```python
from build123d import *

# Parameters (mm, degrees)
EXTRUDE_1_DEPTH     = 50
SKETCH_2_R          = 2
CUT_EXTRUDE_1_DEPTH = 51.670109532


with BuildPart() as part:
    # Эскиз1 → Бобышка-Вытянуть1 (new body)
    with BuildSketch(Plane.XY):
        with BuildLine():
            Line((-3.05, 2.308700651), (-3.05, -4.308700651))
            ThreePointArc((-3.05, -4.308700651), (0, -5.5), (3.05, -4.308700651))
            Line((3.05, -4.308700651), (3.05, 2.308700651))
            ThreePointArc((3.05, 2.308700651), (0, 3.5), (-3.05, 2.308700651))
        make_face()
    extrude(amount=EXTRUDE_1_DEPTH)

    # Эскиз2 → Вырез-Вытянуть1 (cut, through all)
    with BuildSketch(Plane.ZY.offset(3.05)):
        with Locations(Location((46, -1, 0), (0, 0, 270))):
            Circle(SKETCH_2_R)
    extrude(amount=-CUT_EXTRUDE_1_DEPTH, mode=Mode.SUBTRACT)


solid = part.part
```
Design review of the part built by this model. Coordinates are the model's own, in mm. Coordinates: 2 decimals unless noted, no trailing zeros. Write each loop counter-clockwise with the first axis right and the second up, starting at its lowest first coordinate (ties: lowest second). Pieces come first, ordered by that corner, then holes.
1) Insertion check: pin 1 (2 mm diameter, centred on x = 1, z = 11.5, fed in from +Y). The pin has a flat end and moves straight along its axis. Give the tip position at first contact, or say it passes through.
2) Mouldability with a two-part tool opening along Z and no side actions: class faces 1 (the flat face through (0, -1, 50)), 2 (the cylindrical face through (0, -5.5, 24.6)), 3 (the cylindrical face through (-0.043, -1.923, 44.226)) as +Z half, -Z half, draft (parallel to the pull), parting line (faces both ways), or undercut.
3) Add section B-B (z = 46). Write out the cut boundary in (x, y), plus the area to 3 significant figures.
4) Add section A-A (x = 0). Write out the cut boundary in (y, z).
5) To check wall thickness, follow L1, parallel to Z at x = 1.75, y = -1; L2, parallel to Y at x = 1.25, z = 47; L3, parallel to Z at x = 2.5, y = -2.5. State the ranges of each line that lie inside material, in increasing order.
6) Add section C-C (y = -1). Write out the cut boundary in (x, z).
7) Add section D-D (z = 29). Write out the cut boundary in (x, y).
Check result:
1. pin 1: stops at y = 3.5
2. face 1: +Z half
2. face 2: draft
2. face 3: undercut
3. outline: (-3.05, -4.31) arc R4.5 ccw to (3.05, -4.31) - (3.05, -3) - (-3.05, -3) - close; (-3.05, 1) - (3.05, 1) - (3.05, 2.31) arc R4.5 ccw to (-3.05, 2.31) - close
3. area: 25.9 mm2
4. outline: (-5.5, 0) - (3.5, 0) - (3.5, 50) - (-5.5, 50) - close; hole circle Ø4 at (-1, 46)
5. L1: z = 0 to 44, 48 to 50
5. L2: y = -5.32 to -2.73, 0.73 to 3.32
5. L3: z = 0 to 44.68, 47.32 to 50
6. outline: (-3.05, 0) - (3.05, 0) - (3.05, 44) - (-3.05, 44) - close; (-3.05, 48) - (3.05, 48) - (3.05, 50) - (-3.05, 50) - close
7. outline: (-3.05, -4.31) arc R4.5 ccw to (3.05, -4.31) - (3.05, 2.31) arc R4.5 ccw to (-3.05, 2.31) - close
